Part model, mm, in its own coordinate system. Face numbers are marked on the shaded views. A direction names the side the tool comes from. Coordinates: 2 decimals unless noted, no trailing zeros. Order: outer loops, then holes, each group sorted by start corner. A loop starts at its lowest first (then second) coordinate and runs counter-clockwise, first axis right, second up.
from build123d import *

# Parameters (mm, degrees)
F0_W      = 15
F0_H      = 15
F1_DEPTH  = 45
F2_R      = 5
F3_DEPTH  = 45
F4_R      = 7.5
F6_W      = 10
F6_H      = 5
F7_DEPTH  = 45
F8_W      = 7
F8_H      = 2.5
F9_DEPTH  = 45
F10_W     = 15
F10_H     = 5
F11_DEPTH = 8
F12_W     = 15
F12_H     = 5
F13_DEPTH = 8
F14_R     = 1
F15_DEPTH = 45
F16_R     = 2
F17_SIZE  = 0.5


with BuildPart() as f1:
    # F0 (on Front) → F1 (new body)
    with BuildSketch(Plane.XZ):
        with Locations((7.5, 7.5)):
            Rectangle(F0_W, F0_H)
    extrude(amount=-F1_DEPTH)

    # F2 (on face) → F3 (cut)
    with BuildSketch(Plane.XZ):
        with Locations((7.5, 7.5)):
            Circle(F2_R)
    extrude(amount=-F3_DEPTH, mode=Mode.SUBTRACT)

    # F4
    f4_edges = [f1.edges().sort_by_distance(p)[0] for p in [
        (15, 22.5, 15),
    ]]
    fillet(f4_edges, radius=F4_R)

    # F6 (on face) → F7 (join)
    with BuildSketch(Plane.XZ):
        with Locations((5, -2.5)):
            Rectangle(F6_W, F6_H)
    extrude(amount=-F7_DEPTH)

    # F8 (on face) → F9 (cut)
    with BuildSketch(Plane.XZ):
        with Locations((6.5, -1.25)):
            Rectangle(F8_W, F8_H)
    extrude(amount=-F9_DEPTH, mode=Mode.SUBTRACT)

    # F10 (on face) → F11 (join)
    with BuildSketch(Plane(origin=(0, 0, 0), x_dir=(0, -1, 0), z_dir=(-1, 0, 0))):
        with Locations((-7.5, -2.5)):
            Rectangle(F10_W, F10_H)
    extrude(amount=F11_DEPTH)

    # F12 (on face) → F13 (join)
    with BuildSketch(Plane(origin=(0, 0, 0), x_dir=(0, -1, 0), z_dir=(-1, 0, 0))):
        with Locations((-37.5, -2.5)):
            Rectangle(F12_W, F12_H)
    extrude(amount=F13_DEPTH)

    # F14 (on face) → F15 (cut)
    with BuildSketch(Plane(origin=(0, 45, 0), x_dir=(-1, 0, 0), z_dir=(0, 1, 0))):
        with Locations((4, -2.5)):
            Circle(F14_R)
    extrude(amount=-F15_DEPTH, mode=Mode.SUBTRACT)

    # F16
    f16_edges = [f1.edges().sort_by_distance(p)[0] for p in [
        (-8, 37.5, 0),
        (-8, 37.5, -5),
        (-8, 7.5, -5),
        (-8, 7.5, 0),
        (0, 22.5, 15),
    ]]
    fillet(f16_edges, radius=F16_R)

    # F17
    f17_edges = [f1.edges().sort_by_distance(p)[0] for p in [
        (0, 0, 6.5),
        (-3, 0, 0),
        (10, 0, -3.75),
        (6.5, 0, -2.5),
        (3, 0, -1.25),
        (9, 0, 0),
        (2.5, 0, 7.5),
        (-3, 15, -5),
        (-3, 15, -2.5),
        (-3, 0, -2.5),
        (-3, 30, -2.5),
        (2, 0, -5),
        (-7.414214, 45, -4.414214),
        (10, 45, -3.75),
        (6.5, 45, -2.5),
        (3, 45, -1.25),
        (9, 45, 0),
        (2.5, 45, 7.5),
        (15, 45, 3.75),
        (-3, 45, -2.5),
        (15, 22.5, 0),
        (10, 22.5, -5),
        (10, 22.5, -2.5),
        (0, 22.5, -5),
        (4.75, 0, 15),
        (4.75, 45, 15),
        (0.585786, 0, 14.414214),
        (12.803301, 0, 12.803301),
        (15, 0, 3.75),
        (-7.414214, 0, -0.585786),
        (-8, 0, -2.5),
        (-7.414214, 0, -4.414214),
        (0.585786, 45, 14.414214),
        (12.803301, 45, 12.803301),
        (0, 45, 6.5),
        (-3, 45, 0),
        (-7.414214, 45, -0.585786),
        (-8, 45, -2.5),
        (2, 45, -5),
        (-3, 15, 0),
        (-7.414214, 15, -0.585786),
        (-8, 15, -2.5),
        (-7.414214, 15, -4.414214),
        (-3, 30, -5),
        (-3, 30, 0),
        (-7.414214, 30, -0.585786),
        (-8, 30, -2.5),
        (-7.414214, 30, -4.414214),
    ]]
    chamfer(f17_edges, length=F17_SIZE)


solid = f1.part
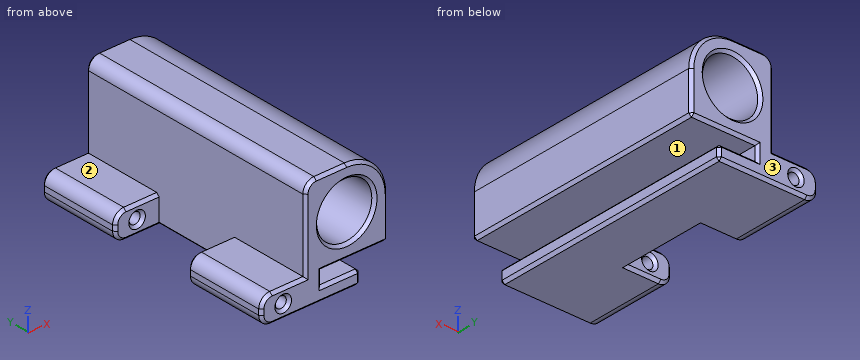
Q1. Cut at C-C on y = 24.5. Write the cut outline in (x, z), and give its area (3 significant figures).
Results list:
outline: (0, -4.5) - (0.5, -5) - (9.5, -5) - (10, -4.5) - (10, -3) - (9.5, -2.5) - (3, -2.5) - (3, 0) - (14.5, 0) - (15, 0.5) - (15, 7.5) arc R7.5 ccw to (7.5, 15) - (2, 15) arc R2 ccw to (0, 13) - close; hole circle Ø10 at (7.5, 7.5)
area: 166 mm2
Q2. Cut at B-B on y = 32. Write the cut outline in (x, z), and give its area (3 significant figures).
Results list:
outline: (-8, -3) arc R2 ccw to (-6, -5) - (9.5, -5) - (10, -4.5) - (10, -3) - (9.5, -2.5) - (3, -2.5) - (3, 0) - (14.5, 0) - (15, 0.5) - (15, 7.5) arc R7.5 ccw to (7.5, 15) - (2, 15) arc R2 ccw to (0, 13) - (0, 0) - (-6, 0) arc R2 ccw to (-8, -2) - close; hole circle Ø2 at (-4, -2.5); hole circle Ø10 at (7.5, 7.5)
area: 201 mm2
Q3. Pin check, flat tips, straight feed: pin 1 Ø9 at (y, z) = (25, 6) entering from -X; pin 2 Ø0.5 at (y, z) = (28, -4) entering from +X; pin 3 Ø2 at (x, y) = (12.5, 10.5) entering from -Z. Stop position of each tip, or through.
Results list:
pin 1: stops at x = 0
pin 2: stops at x = 10
pin 3: stops at z = 0
Q4. Wall check: line 1 along Z through (x, y) = (-4, 10.75); line 2 along Z through (x, y) = (-0.75, 9.5); line 3 along Z through (x, y) = (9.25, 39). Give the ranges that are in metal, low to high.
Results list:
line 1: z = -5 to -3.5, -1.5 to 0
line 2: z = -5 to 0
line 3: z = -5 to -2.5, 0 to 2.82, 12.18 to 14.79
Q5. Which spindle directions (+Z, -Z, +X, -X, +Y, -Y) get a long thin tool onto all of the face, cutting with end or side? Do the marked faces 1, 2 and 3. Say none if no direction does.
Results list:
face 1: +X, +Y, -Y
face 2: +Z, -X, +Y, -Y
face 3: +Z, -Z, +X, -X, +Y
Q6. Cut at A-A on x = -4. Count the separate pieces of the cut face and the enclosed holes in it, and give its area (3 significant figures).
Results list:
separate pieces: 4
enclosed holes: 0
area: 88.0 mm2
